Geometry check sheet. Reference: the model listing, model coordinates, mm. Give positions to 0.01 mm unless a question says otherwise; leave off trailing zeros. Write each loop counter-clockwise with the first axis right and the second up, starting at its lowest first coordinate (ties: lowest second). Pieces come first, ordered by that corner, then holes. Notation, with made-up numbers: (-38, 29) - (2, 29) arc R15 cw to (2, 47) - close; hole circle Ø11 at (26, 85.5). An arc over 180 degrees is marked (long way). Use a Markdown table: item, result.
```python
from build123d import *

# Parameters (mm, degrees)
SKETCH_1_R          = 17.3
SKETCH_1_R_2        = 13.2
EXTRUDE_1_DEPTH     = 2.2
SKETCH_2_R          = 14.394054642
CUT_EXTRUDE_1_DEPTH = 1
CUT_EXTRUDE_2_DEPTH = 1
FILLET_1_R          = 0.5


with BuildPart() as part:
    # 草图1 → 凸台-拉伸1 (new body)
    with BuildSketch(Plane.XY):
        Circle(SKETCH_1_R)
        Circle(SKETCH_1_R_2, mode=Mode.SUBTRACT)
    extrude(amount=EXTRUDE_1_DEPTH)

    # 草图2 → 切除-拉伸1 (cut)
    with BuildSketch(Plane(origin=(0, 0, 0), x_dir=(-1, 0, 0), z_dir=(0, 0, -1))):
        Circle(SKETCH_2_R)
    extrude(amount=-CUT_EXTRUDE_1_DEPTH, mode=Mode.SUBTRACT)

    # 草图3 → 切除-拉伸2 (cut)
    with BuildSketch(Plane(origin=(0, 0, 0), x_dir=(-1, 0, 0), z_dir=(0, 0, -1))):
        with BuildLine():
            Line((-2.642058299, 14.986101169), (-2.863597348, 16.242699714))
            ThreePointArc((-2.863597348, 16.242699714), (0, 16.493195075), (2.863597348, 16.242699714))
            Line((2.863597348, 16.242699714), (2.642058299, 14.986101169))
            ThreePointArc((2.642058299, 14.986101169), (0, 15.217217233), (-2.642058299, 14.986101169))
        make_face()
        with BuildLine():
            Line((10.94607932, 10.571047622), (11.863918269, 11.457439813))
            ThreePointArc((11.863918269, 11.457439813), (9.694456828, 13.343275107), (7.23052043, 14.823800393))
            Line((7.23052043, 14.823800393), (6.671139193, 13.676973429))
            ThreePointArc((6.671139193, 13.676973429), (8.94445587, 12.310987348), (10.94607932, 10.571047622))
        make_face()
        with BuildLine():
            Line((15.069070085, 2.118213179), (16.332625651, 2.295827328))
            ThreePointArc((16.332625651, 2.295827328), (15.685960651, 5.09667757), (14.56282516, 7.742713165))
            Line((14.56282516, 7.742713165), (13.436188256, 7.143706702))
            ThreePointArc((13.436188256, 7.143706702), (14.472433609, 4.702378732), (15.069070085, 2.118213179))
        make_face()
        with BuildLine():
            Line((13.436188256, -7.143706702), (14.56282516, -7.742713165))
            ThreePointArc((14.56282516, -7.742713165), (15.685960651, -5.09667757), (16.332625651, -2.295827328))
            Line((16.332625651, -2.295827328), (15.069070085, -2.118213179))
            ThreePointArc((15.069070085, -2.118213179), (14.472433609, -4.702378732), (13.436188256, -7.143706702))
        make_face()
        with BuildLine():
            Line((6.671139193, -13.676973429), (7.23052043, -14.823800393))
            ThreePointArc((7.23052043, -14.823800393), (9.694456828, -13.343275107), (11.863918269, -11.457439813))
            Line((11.863918269, -11.457439813), (10.94607932, -10.571047622))
            ThreePointArc((10.94607932, -10.571047622), (8.94445587, -12.310987348), (6.671139193, -13.676973429))
        make_face()
        with BuildLine():
            Line((-2.642058299, -14.986101169), (-2.863597348, -16.242699714))
            ThreePointArc((-2.863597348, -16.242699714), (0, -16.493195075), (2.863597348, -16.242699714))
            Line((2.863597348, -16.242699714), (2.642058299, -14.986101169))
            ThreePointArc((2.642058299, -14.986101169), (0, -15.217217233), (-2.642058299, -14.986101169))
        make_face()
        with BuildLine():
            Line((-10.94607932, -10.571047622), (-11.863918269, -11.457439813))
            ThreePointArc((-11.863918269, -11.457439813), (-9.694456828, -13.343275107), (-7.23052043, -14.823800393))
            Line((-7.23052043, -14.823800393), (-6.671139193, -13.676973429))
            ThreePointArc((-6.671139193, -13.676973429), (-8.94445587, -12.310987348), (-10.94607932, -10.571047622))
        make_face()
        with BuildLine():
            Line((-15.069070085, -2.118213179), (-16.332625651, -2.295827328))
            ThreePointArc((-16.332625651, -2.295827328), (-15.685960651, -5.09667757), (-14.56282516, -7.742713165))
            Line((-14.56282516, -7.742713165), (-13.436188256, -7.143706702))
            ThreePointArc((-13.436188256, -7.143706702), (-14.472433609, -4.702378732), (-15.069070085, -2.118213179))
        make_face()
        with BuildLine():
            Line((-13.436188256, 7.143706702), (-14.56282516, 7.742713165))
            ThreePointArc((-14.56282516, 7.742713165), (-15.685960651, 5.09667757), (-16.332625651, 2.295827328))
            Line((-16.332625651, 2.295827328), (-15.069070085, 2.118213179))
            ThreePointArc((-15.069070085, 2.118213179), (-14.472433609, 4.702378732), (-13.436188256, 7.143706702))
        make_face()
        with BuildLine():
            Line((-6.671139193, 13.676973429), (-7.23052043, 14.823800393))
            ThreePointArc((-7.23052043, 14.823800393), (-9.694456828, 13.343275107), (-11.863918269, 11.457439813))
            Line((-11.863918269, 11.457439813), (-10.94607932, 10.571047622))
            ThreePointArc((-10.94607932, 10.571047622), (-8.94445587, 12.310987348), (-6.671139193, 13.676973429))
        make_face()
    extrude(amount=-CUT_EXTRUDE_2_DEPTH, mode=Mode.SUBTRACT)

    # 圆角1
    fillet_1_edges = [part.edges().sort_by_distance(p)[0] for p in [
        (-17.3, 0, 2.2),
    ]]
    fillet(fillet_1_edges, radius=FILLET_1_R)


solid = part.part
```
1) Section check A-A on x = 0. Record the boundary of the cut face in (y, z), then the cut area to 3 significant figures.
Working result:
| item | result |
|---|---|
| outline | (-17.3, 0) - (-16.49, 0) - (-16.49, 1) - (-15.22, 1) - (-15.22, 0) - (-14.39, 0) - (-14.39, 1) - (-13.2, 1) - (-13.2, 2.2) - (-16.8, 2.2) arc R0.5 ccw to (-17.3, 1.7) - close; (13.2, 1) - (14.39, 1) - (14.39, 0) - (15.22, 0) - (15.22, 1) - (16.49, 1) - (16.49, 0) - (17.3, 0) - (17.3, 1.7) arc R0.5 ccw to (16.8, 2.2) - (13.2, 2.2) - close |
| area | 13.0 mm² |
2) Mould release check, pull along X, two halves, no side actions. Record for faces 1 (the flat face through (11.41, 11.02, 0.49)), 2 (the flat face through (-10, -9, 2.2)): pulls with the +X half, pulls with the -X half, needs draft (parallel to the pull), parting line crosses it, or undercut.
Working result:
| item | result |
|---|---|
| face 1 | undercut |
| face 2 | needs draft |
3) Section check C-C on z = 0.6. Count the separate pieces of the cut face and the enclosed holes in it, then the cut area to 3 significant figures.
Working result:
| item | result |
|---|---|
| separate pieces | 1 |
| enclosed holes | 11 |
| area | 219 mm² |
4) Section check B-B on y = 0. Record the boundary of the cut face in (x, z), then the cut area to 3 significant figures.
Working result:
| item | result |
|---|---|
| outline | (-17.3, 0) - (-14.39, 0) - (-14.39, 1) - (-13.2, 1) - (-13.2, 2.2) - (-16.8, 2.2) arc R0.5 ccw to (-17.3, 1.7) - close; (13.2, 1) - (14.39, 1) - (14.39, 0) - (17.3, 0) - (17.3, 1.7) arc R0.5 ccw to (16.8, 2.2) - (13.2, 2.2) - close |
| area | 15.5 mm² |
5) Material ranges on L1, parallel to Y at x = 0, z = 0.4; L2, parallel to Y at x = 0, z = 1.45; L3, parallel to X at y = -4.5, z = 0.45, recorded low to high. Write a range as from..to.
Working result:
| item | result |
|---|---|
| L1 | y = -17.3..-16.49, -15.22..-14.39, 14.39..15.22, 16.49..17.3 |
| L2 | y = -17.3..-13.2, 13.2..17.3 |
| L3 | x = -16.7..-15.87, -14.54..-13.67, 13.67..14.54, 15.87..16.7 |
6) Depth check by flat-ended pin: P1, Ø1, axis at y = 4, z = 1, coming from the +X side; P2, Ø3, axis at x = -13.5, y = -12.5, coming from the +Z side. Enter the tip coordinate at first touch or a pass-through.
Working result:
| item | result |
|---|---|
| P1 | stops at x = 16.94 |
| P2 | stops at z = 2.19 |
